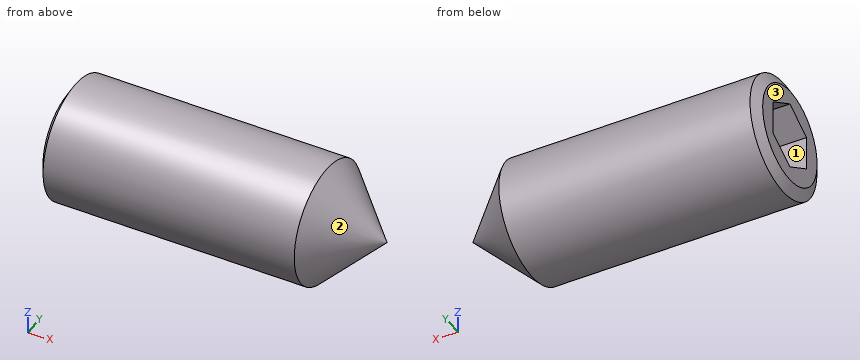
```python
from build123d import *

# Parameters (mm, degrees)
HEX_2_DEPTH = 2.1


with BuildPart() as part:
    # BodySke → BaseBody (revolve)
    with BuildSketch(Plane.XY):
        Polygon((0, 0), (0, 1.2195), (0.161946751, 1.5), (6.505, 1.5), (8, 0.005), (8, 0), align=None)
    revolve(axis=Axis((-12.7, 0, 0), (1, 0, 0)))

    # Sketch2 → Hex 2 (cut)
    with BuildSketch(Plane.ZY):
        Polygon((0.433012702, 0.75), (-0.433012702, 0.75), (-0.866025404, 0), (-0.433012702, -0.75), (0.433012702, -0.75), (0.866025404, 0), align=None)
    extrude(amount=-HEX_2_DEPTH, mode=Mode.SUBTRACT)


solid = part.part
```
Can you work these out from the model? Positions are in its coordinate system, mm. Face numbers are marked on the shaded views. Round coordinates to 2 decimals unless told otherwise and drop trailing zeros. Loops run counter-clockwise (first coordinate to the right, second up) from the corner with the lowest first, then second, coordinate; pieces in that order, holes last. Notation, with made-up numbers: (-13.5, 14) -> (9.5, 14) arc R38 cw to (9.5, 53) -> close; hole circle Ø4 at (45.25, 15.25). An arc over 180 degrees is marked (long way). Answer in a Markdown table with one row per item.
Item 1: We'd pull the mould along Z, two halves only. Please class the marked faces 1, 2 and 3: released by +Z, released by -Z, zero draft, split by the parting line, or undercut.
Answer block:
| item | result |
|---|---|
| face 1 | undercut |
| face 2 | split by the parting line |
| face 3 | zero draft |
Item 2: Will these pins go through, and if not, where does the flat tip stop? P1, Ø1, axis at x = 6.5, y = 1, coming from the -Z side; P2, Ø1.5, axis at y = -1, z = -1, coming from the +X side.
Answer block:
| item | result |
|---|---|
| P1 | z = -1.41 |
| P2 | x = 7.34 |
Item 3: Suppose I cut it at C-C, the plane x = 7.25. List the corners of the cut face in (y, z) for me (3 decimals), plus the area to 3 significant figures.
Answer block:
| item | result |
|---|---|
| outline | circle Ø1.51 at (0, 0) |
| area | 1.79 mm² |
Item 4: Suppose I cut it at B-B, the plane x = 3.25. List the corners of the cut face in (y, z) for me.
Answer block:
| item | result |
|---|---|
| outline | circle Ø3 at (0, 0) |
Item 5: If I drill on probe 1 along Y at (x, z) = (3.25, -1.3); probe 2 along Z at (x, y) = (1, 0.05); probe 3 along Y at (x, z) = (5.5, 0.6), over which ranges is the centre line in solid material (lowest first)?
Answer block:
| item | result |
|---|---|
| probe 1 | -0.75 to 0.75 |
| probe 2 | -1.5 to -0.84, 0.84 to 1.5 |
| probe 3 | -1.37 to 1.37 |
Item 6: Suppose I cut it at A-A, the plane x = 2. List the corners of the cut face in (y, z) for me, plus the area to 3 significant figures.
Answer block:
| item | result |
|---|---|
| outline | circle Ø3 at (0, 0); hole (-0.75, -0.43) -> (0, -0.87) -> (0.75, -0.43) -> (0.75, 0.43) -> (0, 0.87) -> (-0.75, 0.43) -> close |
| area | 5.12 mm² |
